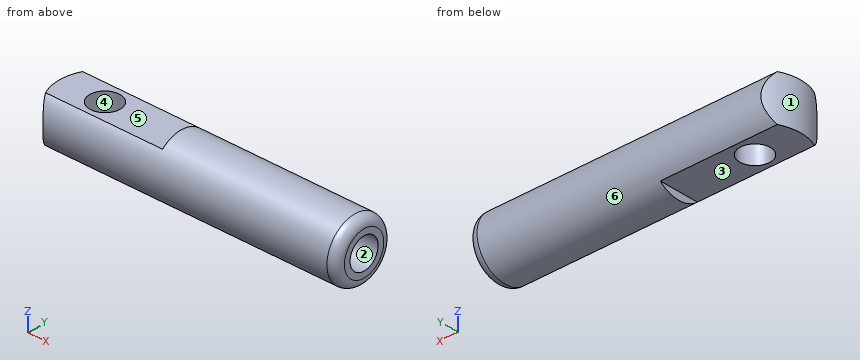
```python
from build123d import *

# Parameters (mm, degrees)
F2_W     = 4
F2_H     = 0.3307065285
F3_DEPTH = 12.5
F4_R     = 0.5
F5_DEPTH = 12.5
F6_R     = 0.3


with BuildPart() as f1:
    # F0 (on Front) → F1 (revolve)
    with BuildSketch(Plane.XZ):
        Polygon((0, 1), (0, 0), (5, 0), (5, 0.5), (10, 0.5), (10, 1), align=None)
    revolve(axis=Axis((2.5, 0, 0), (-1, 0, 0)))

    # F2 (on Front) → F3 (cut, symmetric)
    with BuildSketch(Plane.XZ):
        with Locations((2, 0.9153532643)):
            Rectangle(F2_W, F2_H)
        with Locations((2, -0.9153532643)):
            Rectangle(F2_W, F2_H)
    extrude(amount=F3_DEPTH, both=True, mode=Mode.SUBTRACT)

    # F4 (on Top) → F5 (cut, symmetric)
    with BuildSketch(Plane.XY):
        with BuildLine():
            Line((-0.3413671802, -1.1073484784), (0.495219545, -1.1073484784))
            ThreePointArc((0.495219545, -1.1073484784), (0.1759867726, -0.6948333534), (0.0178750956, -0.197762947))
            ThreePointArc((0.0178750956, -0.197762947), (0.0047393487, 0), (0.0178750956, 0.197762947))
            ThreePointArc((0.0178750956, 0.197762947), (0.1759867726, 0.6948333534), (0.495219545, 1.1073484784))
            Line((0.495219545, 1.1073484784), (-0.3413671802, 1.1073484784))
            Line((-0.3413671802, 1.1073484784), (-0.3413671802, 0))
            Line((-0.3413671802, 0), (-0.3413671802, -1.1073484784))
        make_face()
        with Locations((1.5, 0)):
            Circle(F4_R)
    extrude(amount=F5_DEPTH, both=True, mode=Mode.SUBTRACT)

    # F6
    f6_edges = [f1.edges().sort_by_distance(p)[0] for p in [
        (10, 0, -1),
    ]]
    fillet(f6_edges, radius=F6_R)


solid = f1.part
```
The listing builds one solid part. Answer for the finished solid, in the listing's coordinates (mm). Face numbers are marked on the shaded views. A direction names the side the tool comes from. Coordinates: 2 decimals unless noted, no trailing zeros. Write each loop counter-clockwise with the first axis right and the second up, starting at its lowest first coordinate (ties: lowest second). Pieces come first, ordered by that corner, then holes. Notation, with made-up numbers: (45, 9.5) -> (98, 9.5) arc R20 ccw to (98, 28.5) -> close; hole circle Ø2 at (4, 83). An arc over 180 degrees is marked (long way). Write each question's results on one line, items separated by ' | '. Start each with the question number.
1) Flat-ended cylindrical pins translate along their axes: pin 1 Ø1.1 at (x, y) = (1.5, 0) entering from -Z; pin 2 Ø1.1 at (x, y) = (1.5, 0) entering from +Z. Find the tip coordinate at first contact, or state that the pin passes through.
2) Straight lines are drawn through the part: probe 1 along Y at (x, z) = (8.95, 0); probe 2 along Z at (x, y) = (3.75, 0.4); probe 3 along X at (y, z) = (0.3, 0.7). For each, find the intervals that lie inside material, in ascending order.
3) For a pull along Y with two mould halves and no side action, classify the marked faces 4, 5 and 6 as +Y half, -Y half, draft (parallel to the pull), parting line (faces both ways), or undercut.
4) A cutting plane is placed at C-C (y = 0). Determine the outline of the cut face in (x, z).
5) A tool of negligible diameter and unlimited length cuts with its end or side. For the marked faces 1, 2 and 3, from which of +Z, -Z, +X, -X, +Y, -Y can it reach the whole face along a straight path? Write none if from no direction.
6) A cutting plane is placed at B-B (z = 0). Determine the outline of the cut face in (x, y).
7) A cutting plane is placed at A-A (x = 1.5). Determine the outline of the cut face in (y, z), then the cut area to 3 significant figures.
8) A cutting plane is placed at D-D (x = 3). Determine the outline of the cut face in (y, z), then the cut area to 3 significant figures.
Values follow:
1) pin 1: z = -0.75 | pin 2: z = 0.75
2) probe 1: -1 to -0.5, 0.5 to 1 | probe 2: -0.75 to 0.75 | probe 3: 0.04 to 1.1, 1.9 to 9.99
3) face 4: undercut | face 5: draft | face 6: parting line
4) outline: (0, -0.75) -> (1, -0.75) -> (1, 0.75) -> (0, 0.75) -> close; (2, -0.75) -> (4, -0.75) -> (4, -1) -> (9.7, -1) arc R0.3 ccw to (10, -0.7) -> (10, -0.5) -> (5, -0.5) -> (5, 0.5) -> (10, 0.5) -> (10, 0.7) arc R0.3 ccw to (9.7, 1) -> (4, 1) -> (4, 0.75) -> (2, 0.75) -> close
5) face 1: +Z, -Z, -X | face 2: +X | face 3: -Z, -X, +Y, -Y
6) outline: (0.39, -1) -> (9.7, -1) arc R0.3 ccw to (10, -0.7) -> (10, -0.5) -> (5, -0.5) -> (5, 0.5) -> (10, 0.5) -> (10, 0.7) arc R0.3 ccw to (9.7, 1) -> (0.39, 1) arc R1.5 ccw to start; hole circle Ø1 at (1.5, 0)
7) outline: (-0.66, -0.75) -> (-0.5, -0.75) -> (-0.5, 0.75) -> (-0.66, 0.75) arc R1 ccw to start; (0.5, -0.75) -> (0.66, -0.75) arc R1 ccw to (0.66, 0.75) -> (0.5, 0.75) -> close | area: 1.19 mm²
8) outline: (-0.66, -0.75) -> (0.66, -0.75) arc R1 ccw to (0.66, 0.75) -> (-0.66, 0.75) arc R1 ccw to start | area: 2.69 mm²
